Work out the finished part from the listing and answer in its coordinate system (mm). Face numbers are marked on the shaded views. A direction names the side the tool comes from. Give positions to 0.01 mm unless a question says otherwise; leave off trailing zeros. Loops run counter-clockwise (first coordinate to the right, second up) from the corner with the lowest first, then second, coordinate; pieces in that order, holes last.
from build123d import *

# Parameters (mm, degrees)
BOSS_EXTRUDE3_DEPTH  = 42.5
SKETCH5_3_R          = 70
BOSS_EXTRUDE4_DEPTH  = 49
SKETCH5_6_R          = 70
BOSS_EXTRUDE11_DEPTH = 50
FILLET5_R            = 20
SKETCH6_R            = 12
CUT_EXTRUDE1_DEPTH   = 112
CUT_EXTRUDE2_DEPTH   = 151


with BuildPart() as part:
    # Sketch5 → Boss-Extrude3 (new, symmetric)
    with BuildSketch(Plane(origin=(0, 0, 0), x_dir=(1, 0, 0), z_dir=(0, 1, 0))):
        with BuildLine():
            ThreePointArc((215.042236358, -33.742230992), (251.167097159, -58.991268991), (265.042236358, -100.824270317))
            ThreePointArc((265.042236358, -100.824270317), (251.167097159, -142.657271644), (215.042236358, -167.906309642))
            add(Edge.make_bspline(
                [(215.042236358, -167.906309642), (445.042236358, -134.071536156), (675.042236358, -167.906309642)],
                knots=[0, 0, 0, 1, 1, 1], degree=2))
            ThreePointArc((675.042236358, -167.906309642), (625.042236358, -100.824270317), (675.042236358, -33.742230992))
            add(Edge.make_bspline(
                [(215.042236358, -33.742230992), (445.042236358, -67.577004479), (675.042236358, -33.742230992)],
                knots=[0, 0, 0, 1, 1, 1], degree=2))
        make_face()
    extrude(amount=BOSS_EXTRUDE3_DEPTH, both=True)

    # Sketch5<3> → Boss-Extrude4 (add, symmetric)
    with BuildSketch(Plane(origin=(0, 0, 0), x_dir=(1, 0, 0), z_dir=(0, 1, 0))):
        with Locations(Location((195.042236358, -100.824270317, 0), (0, 0, 270))):
            Circle(SKETCH5_3_R)
    extrude(amount=BOSS_EXTRUDE4_DEPTH, both=True)

    # Sketch5<6> → Boss-Extrude11 (add, symmetric)
    with BuildSketch(Plane(origin=(0, 0, 0), x_dir=(1, 0, 0), z_dir=(0, 1, 0))):
        with Locations(Location((695.042236358, -100.824270317, 0), (0, 0, 270))):
            Circle(SKETCH5_6_R)
    extrude(amount=BOSS_EXTRUDE11_DEPTH, both=True)

    # Fillet5
    fillet5_edges = [part.edges().sort_by_distance(p)[0] for p in [
        (445.042236357, 42.5, 150.988922899),
        (445.042236357, 42.5, 50.659617736),
        (445.042236357, -42.5, 150.988922899),
        (445.042236357, -42.5, 50.659617736),
    ]]
    fillet(fillet5_edges, radius=FILLET5_R)

    # Sketch6 → Cut-Extrude1 (cut)
    with BuildSketch(Plane(origin=(0, -50, 0), x_dir=(1, 0, 0), z_dir=(0, 1, 0))):
        with Locations(Location((195.042236357, -100.824270318, 0), (0, 0, 270))):
            Circle(SKETCH6_R)
    extrude(amount=CUT_EXTRUDE1_DEPTH, mode=Mode.SUBTRACT)

    # Sketch10 → Cut-Extrude2 (cut)
    with BuildSketch(Plane.XZ.offset(50)):
        with BuildLine():
            Line((707.431750575, 96.887274325), (692.978208818, 87.989170384))
            ThreePointArc((692.978208818, 87.989170384), (688.226960704, 111.894591803), (707.431750575, 96.887274325))
        make_face()
    extrude(amount=-CUT_EXTRUDE2_DEPTH, mode=Mode.SUBTRACT)


solid = part.part
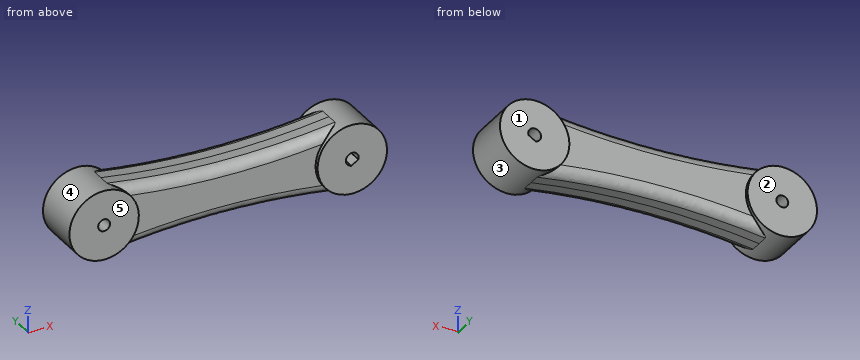
Item 1: Find section A-A, the plane x = 702. Write down the section's boundary in (y, z).
Item 2: Consider line 1 (X direction, y = 11.5, z = 110); line 2 (Y direction, x = 344.5, z = 123); line 3 (Z direction, x = 175, y = 36). Determine where each line is inside the solid, lowest interval first.
Item 3: Find section B-B, the plane y = -34. Give the number of separate pieces and of enclosed holes in the cut face, plus the area to 3 significant figures.
Item 4: Find section D-D, the plane x = 175.5. Write down the section's boundary in (y, z), plus the area to 3 significant figures.
Item 5: Determine the mould class of the marked faces 3, 4 and 5 for opening direction X: released by +X, released by -X, zero draft, split by the parting line, or undercut.
Item 6: For the marked faces 1 and 2, determine the directions among +Z, -Z, +X, -X, +Y, -Y from which every point of the face is accessible in a straight line to the end or side of a thin tool.
Item 7: Flat-ended cylindrical pins translate along their axes: pin 1 Ø5 at (y, z) = (-35.5, 136.5) entering from +X; pin 2 Ø12 at (y, z) = (20.5, 55.5) entering from -X; pin 3 Ø6 at (y, z) = (-29.5, 48) entering from +X. Find the tip coordinate at first contact, or state that the pin passes through.
Ans:
1. outline: (-50, 31.17) - (50, 31.17) - (50, 93.54) - (-50, 93.54) - close; (-50, 111.81) - (50, 111.81) - (50, 170.48) - (-50, 170.48) - close
2. line 1: x = 125.65 to 187.31, 202.78 to 685.83, 704.25 to 764.44
2. line 2: y = -42.5 to 42.5
2. line 3: z = 33.75 to 167.89
3. separate pieces: 1
3. enclosed holes: 2
3. area: 68,100 mm2
4. outline: (-49, 33.61) - (49, 33.61) - (49, 168.04) - (-49, 168.04) - close
4. area: 13,200 mm2
5. face 3: undercut
5. face 4: undercut
5. face 5: zero draft
6. face 1: +Z, -Z, +X, -X, +Y
6. face 2: +Z, -Z, -X, +Y
7. pin 1: stops at x = 756.68
7. pin 2: stops at x = 137.13
7. pin 3: stops at x = 744.21
